Work out the finished part from the listing and answer in its coordinate system (mm). A direction names the side the tool comes from. Give positions to 0.01 mm unless a question says otherwise; leave off trailing zeros. Order: outer loops, then holes, each group sorted by start corner. A loop starts at its lowest first (then second) coordinate and runs counter-clockwise, first axis right, second up.
```python
from build123d import *

# Parameters (mm, degrees)
BASE_EXTRUDE_DEPTH = 3


with BuildPart() as part:
    # Sketch1 → Base-Extrude (new body)
    with BuildSketch(Plane.XY):
        with BuildLine():
            Line((-1361.676742431, 33.692843094), (-1355.157111394, 33.692843094))
            Line((-1355.157111394, 33.692843094), (-1355.157111394, 36.692843094))
            Line((-1355.157111394, 36.692843094), (-1361.676742431, 36.692843094))
            ThreePointArc((-1361.676742431, 36.692843094), (-1363.682913665, 43.843214905), (-1361.676742431, 50.993586716))
            ThreePointArc((-1361.676742431, 50.993586716), (-1351.674443371, 53.537029915), (-1341.672144311, 50.993586716))
            Line((-1341.672144311, 50.993586716), (-1341.672144311, 50.692843094))
            Line((-1341.672144311, 50.692843094), (-1351.065792881, 50.692843094))
            Line((-1351.065792881, 50.692843094), (-1351.065792881, 47.692843094))
            Line((-1351.065792881, 47.692843094), (-1344.113445951, 47.692843094))
            ThreePointArc((-1344.113445951, 47.692843094), (-1333.95450385, 35.192843094), (-1344.113445951, 22.692843094))
            Line((-1344.113445951, 22.692843094), (-1351.065792881, 22.692843094))
            Line((-1351.065792881, 22.692843094), (-1351.065792881, 19.692843094))
            Line((-1351.065792881, 19.692843094), (-1341.672144311, 19.692843094))
            Line((-1341.672144311, 19.692843094), (-1341.672144311, 19.392099471))
            ThreePointArc((-1341.672144311, 19.392099471), (-1351.674443371, 16.848656272), (-1361.676742431, 19.392099471))
            ThreePointArc((-1361.676742431, 19.392099471), (-1363.682913665, 26.542471282), (-1361.676742431, 33.692843094))
        make_face()
    extrude(amount=BASE_EXTRUDE_DEPTH)


solid = part.part
```
1. The part is cut by section A-A (x = -1346.75). Write down the section's boundary in (y, z).
Findings below:
outline: (17.44, 0) - (19.69, 0) - (19.69, 3) - (17.44, 3) - close; (22.69, 0) - (47.69, 0) - (47.69, 3) - (22.69, 3) - close; (50.69, 0) - (52.95, 0) - (52.95, 3) - (50.69, 3) - close
2. The part is cut by section D-D (x = -1343). Write down the section's boundary in (y, z).
Findings below:
outline: (18.73, 0) - (19.69, 0) - (19.69, 3) - (18.73, 3) - close; (22.98, 0) - (47.41, 0) - (47.41, 3) - (22.98, 3) - close; (50.69, 0) - (51.66, 0) - (51.66, 3) - (50.69, 3) - close
3. The mould has two halves that part along Y. Classify faces 1 (the face through (-1363.683, 43.738, 1.479)), 2 (the face through (-1351.53, 16.85, 1.48)), 3 (the face through (-1351.82, 53.537, 1.479)): pulls with the +Y half, pulls with the -Y half, needs draft (parallel to the pull), parting line crosses it, or undercut.
Findings below:
face 1: undercut
face 2: pulls with the -Y half
face 3: pulls with the +Y half
4. Which of the six approach directions +Z, -Z, +X, -X, +Y, -Y give full straight-line access (tool end or side, diameter ignored) to faces 4 (the face through (-1355.157, 35, 1)), 5 (the face through (-1349, 35, 3)), 6 (the face through (-1348, 47.693, 1))?
Findings below:
face 4: +Z, -Z, -X
face 5: +Z, +X, -X, +Y, -Y
face 6: +Z, -Z, +X
5. Given P1, Ø0.9, axis at y = 20.5, z = 1, coming from the +X side; P2, Ø0.9, axis at x = -1345, z = 1.5, coming from the +Y side; P3, Ø1.5, axis at x = -1358, z = 2, coming from the +Y side; P4, Ø12, axis at x = -1352.5, y = 23.5, coming from the -Z side, each flat-ended and moving along its own axis, determine where each tip first touches the part or whether it passes through.
Findings below:
P1: stops at x = -1351.07
P2: stops at y = 52.59
P3: stops at y = 52.78
P4: stops at z = 0
6. The part is cut by section C-C (x = -1360). Write down the section's boundary in (y, z).
Findings below:
outline: (18.57, 0) - (33.69, 0) - (33.69, 3) - (18.57, 3) - close; (36.69, 0) - (51.81, 0) - (51.81, 3) - (36.69, 3) - close
7. Straight lines are drawn through the part: probe 1 along Y at (x, z) = (-1342, 1.55); probe 2 along Y at (x, z) = (-1351.75, 0.9); probe 3 along Y at (x, z) = (-1360, 0.9). For each, find the intervals that lie inside material, in ascending order.
Findings below:
probe 1: y = 19.22 to 19.69, 23.33 to 47.06, 50.69 to 51.17
probe 2: y = 16.85 to 53.54
probe 3: y = 18.57 to 33.69, 36.69 to 51.81
8. The part is cut by section B-B (z = 2.1). Write down the section's boundary in (x, y), then the cut area to 3 significant figures.
Findings below:
outline: (-1361.68, 19.39) arc R20.94 ccw to (-1341.67, 19.39) - (-1341.67, 19.69) - (-1351.07, 19.69) - (-1351.07, 22.69) - (-1344.11, 22.69) arc R12.77 ccw to (-1344.11, 47.69) - (-1351.07, 47.69) - (-1351.07, 50.69) - (-1341.67, 50.69) - (-1341.67, 50.99) arc R20.94 ccw to (-1361.68, 50.99) arc R13.75 ccw to (-1361.68, 36.69) - (-1355.16, 36.69) - (-1355.16, 33.69) - (-1361.68, 33.69) arc R13.75 ccw to start
area: 793 mm2
